Autodesk Inventor part; units mm, degrees
ref_plane "YZ Plane" through (0, 0, 0) normal (1, 0, 0) x (0, 1, 0)
ref_plane "XZ Plane" through (0, 0, 0) normal (0, 1, 0) x (-1, 0, 0)
ref_plane "XY Plane" through (0, 0, 0) normal (0, 0, 1) x (1, 0, 0)
sketch "スケッチ1" plane through (0, 0, 0) normal (0, 0, 1) x (1, 0, 0)
  line L0 (0, 0) -> (0, -60) construction
  arc A0 (0, -4) -> (3.9768, -0.4299) centre (0, 0) ccw construction
  arc A1 (0, -55) -> (-4.9993, -59.9167) centre (0, -60) ccw construction
  arc A2 (3.9768, -0.4299) -> (4.9505, -59.2985) centre (240.1879, -25.9652) ccw
  arc A3 (-3.9994, 0.0667) -> (0, -4) centre (0, 0) ccw construction
  arc A4 (3.9768, -0.4299) -> (4, 0) centre (0, 0) ccw
  arc A5 (4.9505, -59.2985) -> (0, -55) centre (0, -60) ccw construction
  arc A6 (-4.9993, -59.9167) -> (4.9505, -59.2985) centre (0, -60) ccw
  line L1 (-3.9994, 0.0667) -> (-4.9993, -59.9167)
  line L2 (2.6336, -22.0054) -> (2.3154, -41.0967) construction
  circle A7 centre (0, 0) radius 2 construction
  line L3 (-1.12, 3.84) -> (1.76, 4.68)
  line L4 (4, 3) -> (4, 0)
  arc A8 (4, 3) -> (1.76, 4.68) centre (2.25, 3) ccw
  circle A9 centre (2.25, 3) radius 1 construction
  arc A10 (-1.12, 3.84) -> (-3.9994, 0.0667) centre (0, 0) ccw
  arc A11 (4, 0) -> (-1.12, 3.84) centre (0, 0) ccw construction
  circle A12 centre (2.25, 3) radius 1.75 construction
  line L5 (-0.3242, -5.7627) -> (0, 0) construction
  circle A13 centre (-0.3242, -5.7627) radius 3.7718 construction
  circle A14 centre (0, -60) radius 2 construction
  circle A15 centre (0, -60) radius 3.5 construction
  line L6 (0, -60) -> (2.4749, -62.4749) construction
  circle A16 centre (-0.3611, -53.4798) radius 4.5302 construction
  dimension "d26" = 7
  dimension "d0" = 60
  dimension "d1" = 4
  dimension "d2" = 5
  dimension "d14" = 7
  dimension "d15" = 4
  dimension "d16" = 1.75
  dimension "d17" = 2
  dimension "d25" = 4
  dimension "d27" = 45
extrude "押し出し1" add sketch "スケッチ1" along normal blind 2
hole "穴1" at (0, 0, 0) at (0, -60, 0) direction (0, 0, 1) diameter 4 end through all
hole "穴2" at (-0.3611, -53.4798, 0) at (2.4749, -62.4749, 0) direction (0, 0, 1) diameter 1.4 end through all countersink diameter 2.5 countersink angle 90
sketch "スケッチ2" plane through (0, 0, 2) normal (0, 0, 1) x (1, 0, 0)
  point P0 (0, 0)
  point P1 (2.25, 3)
  point P2 (-0.3242, -5.7627)
hole "穴4" at (2.25, 3, 2) at (-0.3242, -5.7627, 2) direction (0, 0, -1) diameter 1.4 end through all countersink diameter 2.5 countersink angle 90
properties part number "COXA_ROLL_LONG-LINK"
Here's how the part is built. I have some questions about the finished solid (model axes, mm). Coordinates: 2 decimals unless noted, no trailing zeros. Order: outer loops, then holes, each group sorted by start corner. A loop starts at its lowest first (then second) coordinate and runs counter-clockwise, first axis right, second up.
Item 1: If we section it at A-A on y = -42: List the corners of the cut face in (x, z) for me, plus the area to 3 significant figures.
Result sheet:
outline: (-4.7, 0) - (3.14, 0) - (3.14, 2) - (-4.7, 2) - close
area: 15.7 mm2
Item 2: I need wall thicknesses on line 1 (Y direction, x = 0, z = 0.7); line 2 (Y direction, x = 0.5, z = 0.55); line 3 (Y direction, x = 1.5, z = 1). Which ranges of each line are inside material? Lowest first, please.
Result sheet:
line 1: y = -65 to -62, -58 to -54.08, -52.88 to -6.38, -5.14 to -2, 2 to 4.17
line 2: y = -64.97 to -61.94, -58.06 to -1.94, 1.94 to 4.31
line 3: y = -64.77 to -61.32, -58.68 to -1.32, 1.32 to 4.6
Item 3: If we mould it in two halves opening along Y, with no side actions, what happens to faces 1 (the face through (0.3, 4.254, 0.986)), 2 (the face through (4, 2, 1)), 3 (the face through (-0.39, -54.18, 1.29))? For each: +Y half, -Y half, draft (parallel to the pull), parting line (faces both ways), or undercut.
Result sheet:
face 1: +Y half
face 2: draft
face 3: undercut
Item 4: For P1, Ø1.8, axis at x = 2.47, y = -62.47, coming from the -Z side; P2, Ø0.8, axis at x = -0.36, y = -53.48, coming from the -Z side (3 decimals); P3, Ø1.6, axis at x = 2.25, y = 3, coming from the +Z side; P4, Ø1, axis at y = 1, z = 1.5, coming from the +X side, each with a flat end and sliding along its axis, tell me the tip position at first contact or that it passes through.
Result sheet:
P1: stops at z = 0.34
P2: passes through
P3: stops at z = 1.55
P4: stops at x = 4
Item 5: If we section it at B-B on y = -12: List the corners of the cut face in (x, z) for me, plus the area to 3 significant figures.
Result sheet:
outline: (-4.2, 0) - (3.01, 0) - (3.01, 2) - (-4.2, 2) - close
area: 14.4 mm2
